Print and shaded views of the part. All mm, measured from the part's lowest x, y and z. Round coordinates to 2 decimals unless told otherwise and drop trailing zeros. Loops run counter-clockwise (first coordinate to the right, second up) from the corner with the lowest first, then second, coordinate; pieces in that order, holes last. Notation, with made-up numbers: (22, 19) - (50, 19) arc R13 ccw to (50, 35) - close; hole circle Ø5 at (76.25, 78). An arc over 180 degrees is marked (long way). Use one line per item in the form item = value.
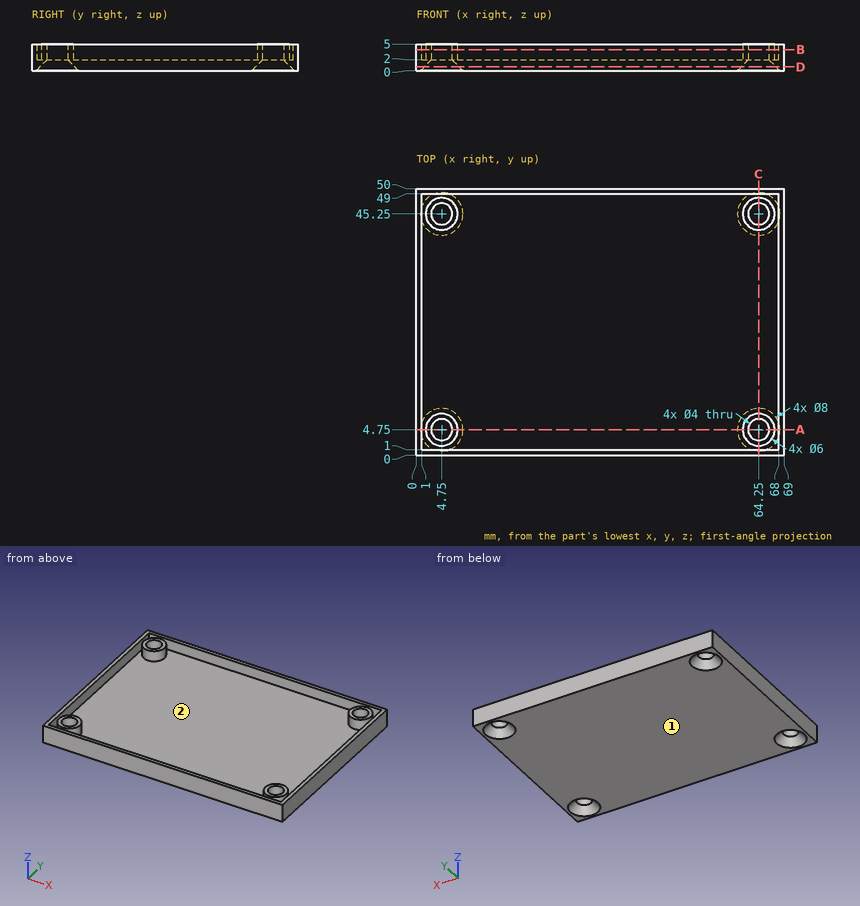
1. Wall check: probe 1 along Y at (x, z) = (64.25, 3.25); probe 2 along Y at (x, z) = (20.5, 2.8); probe 3 along X at (y, z) = (30, 4.5). Give the ranges that are in metal, low to high.
Geometry check:
probe_1 = 0 to 1, 1.75 to 2.75, 6.75 to 7.75, 42.25 to 43.25, 47.25 to 48.25, 49 to 50
probe_2 = 0 to 1, 49 to 50
probe_3 = 0 to 1, 68 to 69
2. Cut at B-B, the plane z = 3.95. Give the number of separate pieces and of enclosed holes in the cut face, plus the area to 3 significant figures.
Geometry check:
separate_pieces = 5
enclosed_holes = 5
area = 297 mm^2
3. Flat gauge pins, fed straight in: pin 1 (2 mm diameter, centred on x = 25, y = 23.5, fed in from +Z); pin 2 (3.5 mm diameter, centred on x = 64.25, y = 4.75, fed in from +Z); pin 3 (6.5 mm diameter, centred on x = 4.75, y = 4.75, fed in from -Z). Where does each tip first touch, or does it go through?
Geometry check:
pin_1 = 2
pin_2 = through
pin_3 = 0.75
4. Cut at D-D, the plane z = 0.7. Give the cut face in (x, y).
Geometry check:
outline = (0, 0) - (69, 0) - (69, 50) - (0, 50) - close; hole circle Ø6.6 at (4.75, 4.75); hole circle Ø6.6 at (4.75, 45.25); hole circle Ø6.6 at (64.25, 4.75); hole circle Ø6.6 at (64.25, 45.25)
5. Cut at C-C, the plane x = 64.25. Give the cut face in (y, z), plus the area to 3 significant figures.
Geometry check:
outline = (0, 0) - (0.75, 0) - (2.75, 2) - (2.75, 5) - (1.75, 5) - (1.75, 2) - (1, 2) - (1, 5) - (0, 5) - close; (6.75, 2) - (8.75, 0) - (41.25, 0) - (43.25, 2) - (43.25, 5) - (42.25, 5) - (42.25, 2) - (7.75, 2) - (7.75, 5) - (6.75, 5) - close; (47.25, 2) - (49.25, 0) - (50, 0) - (50, 5) - (49, 5) - (49, 2) - (48.25, 2) - (48.25, 5) - (47.25, 5) - close
area = 94.0 mm^2
6. Cut at A-A, the plane y = 4.75. Give the cut face in (x, z).
Geometry check:
outline = (0, 0) - (0.75, 0) - (2.75, 2) - (2.75, 5) - (1.75, 5) - (1.75, 2) - (1, 2) - (1, 5) - (0, 5) - close; (6.75, 2) - (8.75, 0) - (60.25, 0) - (62.25, 2) - (62.25, 5) - (61.25, 5) - (61.25, 2) - (7.75, 2) - (7.75, 5) - (6.75, 5) - close; (66.25, 2) - (68.25, 0) - (69, 0) - (69, 5) - (68, 5) - (68, 2) - (67.25, 2) - (67.25, 5) - (66.25, 5) - close
7. Pull direction X, two halves, no side cores. Call the marked faces 1 and 2: +X half, -X half, draft (parallel to the pull), parting line (faces both ways), or undercut.
Geometry check:
face_1 = draft
face_2 = undercut
